from build123d import *

# Parameters (mm, degrees)
SKETCH_1_R               = 20
EXTRUDE_2_DEPTH          = 100
EXTRUDE_3_DEPTH          = 20
SKETCH_3_R               = 10.544762533
EXTRUDE_4_DEPTH          = 20
SKETCH_4_R               = 8
EXTRUDE_5_DEPTH          = 70
EXTRUDE_START            = 100
SKETCH_5_R               = 20
EXTRUDE_6_DEPTH          = 100
EXTRUDE_8_DEPTH          = 20
SKETCH_7_R               = 10.548482156
EXTRUDE_9_DEPTH          = 20
SKETCH_8_R               = 8
EXTRUDE_10_DEPTH         = 70
CUT_EXTRUDE_1_REACH      = 231.885
CUT_EXTRUDE_1_END_RADIUS = 20


with BuildPart() as part:
    # 草图1 → 凸台-拉伸2 (new body)
    with BuildSketch(Plane.XY):
        Circle(SKETCH_1_R)
    extrude(amount=EXTRUDE_2_DEPTH)

    # 草图2 → 凸台-拉伸3 (add)
    with BuildSketch(Plane.XY.offset(100)):
        Polygon((-20, 0), (-10.544762533, -101.307170503), (10.544762533, -101.307170503), (20, 0), align=None)
    extrude(amount=-EXTRUDE_3_DEPTH)

    # 草图3 → 凸台-拉伸4 (add, symmetric)
    with BuildSketch(Plane.XY.offset(100)):
        with Locations((0, -101.307170503)):
            Circle(SKETCH_3_R)
    extrude(amount=EXTRUDE_4_DEPTH, both=True)

    # 草图4 → 凸台-拉伸5 (add)
    with BuildSketch(Plane.XY.offset(120)):
        with Locations((0, -101.307170503)):
            Circle(SKETCH_4_R)
    extrude(amount=EXTRUDE_5_DEPTH)

    # 草图5 → 凸台-拉伸6 (add)
    with BuildSketch(Plane(origin=(0, 0, 0), x_dir=(-1, 0, 0), z_dir=(0, 0, -1)).offset(EXTRUDE_START)):
        Circle(SKETCH_5_R)
    extrude(amount=-EXTRUDE_6_DEPTH)

    # 草图6 → 凸台-拉伸8 (add)
    with BuildSketch(Plane(origin=(0, 0, -100), x_dir=(-1, 0, 0), z_dir=(0, 0, -1))):
        Polygon((20, 0), (10.548482156, 101.307517591), (-10.548482156, 101.307517591), (-20, 0), align=None)
    extrude(amount=-EXTRUDE_8_DEPTH)

    # 草图7 → 凸台-拉伸9 (add, symmetric)
    with BuildSketch(Plane(origin=(0, 0, -100), x_dir=(-1, 0, 0), z_dir=(0, 0, -1))):
        with Locations((0, 101.307517591)):
            Circle(SKETCH_7_R)
    extrude(amount=EXTRUDE_9_DEPTH, both=True)

    # 草图8 → 凸台-拉伸10 (add)
    with BuildSketch(Plane(origin=(0, 0, -120), x_dir=(-1, 0, 0), z_dir=(0, 0, -1))):
        with Locations((0, 101.307517591)):
            Circle(SKETCH_8_R)
    extrude(amount=EXTRUDE_10_DEPTH)

    # 切除-拉伸1: up to this cylinder (the profile starts inside it)
    cut_extrude_1_end = Plane(origin=(0, 0, 0), z_dir=(0, 0, -1)) * Cylinder(CUT_EXTRUDE_1_END_RADIUS, 504.77, mode=Mode.PRIVATE)
    # 草图9 → 切除-拉伸1 (cut, up to the surface)
    with BuildSketch(Plane(origin=(0, -16, 0), x_dir=(1, 0, 0), z_dir=(0, 1, 0)), mode=Mode.PRIVATE) as cut_extrude_1_sk1:
        with BuildLine():
            Line((6, -8), (6, 8))
            ThreePointArc((6, 8), (0, 14), (-6, 8))
            Line((-6, 8), (-6, -8))
            ThreePointArc((-6, -8), (0, -14), (6, -8))
        make_face()
    cut_extrude_1_tool1 = extrude(cut_extrude_1_sk1.sketch, amount=-CUT_EXTRUDE_1_REACH, mode=Mode.PRIVATE) & cut_extrude_1_end
    add(cut_extrude_1_tool1.solids().sort_by_distance((0, -16, 0))[0], mode=Mode.SUBTRACT)


solid = part.part
Source: CAD feature listing. Evaluate the final solid. Frame: model axes, mm. A direction names the side the tool comes from. Give positions to 0.01 mm unless a question says otherwise; leave off trailing zeros. Write each loop counter-clockwise with the first axis right and the second up, starting at its lowest first coordinate (ties: lowest second). Pieces come first, ordered by that corner, then holes. Notation, with made-up numbers: (-15.75, -0.5) -> (26.25, -0.5) arc R27 ccw to (26.25, 23.5) -> close; hole circle Ø2 at (24, 67.25). An arc over 180 degrees is marked (long way). Return JSON: item names as keys, results as strings. Group by question number.
1. Mould query, pull axis Z, two halves, no side actions, for faces 1 (the face through (0, -16, 0)), 2 (the face through (-2, -93, 120)), 3 (the face through (8, 104, -120)), 4 (the face through (1.373, 111.766, -104.724)). Classes: +Z half, -Z half, draft (parallel to the pull), parting line (faces both ways), or undercut.
2. Material intervals for line 1 (Z direction, x = 2, y = 38); line 2 (Y direction, x = 17, z = -7.5); line 3 (Z direction, x = 11, y = -48), sorted ascending. Write a range as from..to.
3. Pin query (flat end, axial travel): pin 1 Ø20 at (x, y) = (-1.5, 56.5) entering from -Z; pin 2 Ø10 at (x, z) = (13.5, 42.5) entering from -Y; pin 3 Ø2 at (x, y) = (3, 79.5) entering from +Z. Return the tip coordinate at first contact, or that it passes through.
4. Access query for faces 5 (the face through (1.04, 109.24, -154.51)), 6 (the face through (4.87, -110.66, 104.72)), 7 (the face through (0, 101, -190)). Directions: +Z, -Z, +X, -X, +Y, -Y. A direction counts if a zero-diameter tool reaches every point of the face in a straight line with its end or side. Return the directions, or none.
5. Section C-C, the plane y = -74. Output: boundary loops of the cut face in (x, z).
6. Section D-D, the plane z = 52. Output: boundary loops of the cut face in (x, y).
7. Section A-A, the plane x = 2. Output: boundary loops of the cut face in (y, z).
8. Section B-B, the plane z = -88.5. Output: boundary loops of the cut face in (x, y).
Determined:
{
 "1": {"face 1": "undercut", "face 2": "+Z half", "face 3": "-Z half", "face 4": "draft"},
 "2": {"line 1": "z = -100..-80", "line 2": "y = -10.54..10.54", "line 3": "z = 80..100"},
 "3": {"pin 1": "stops at z = -100", "pin 2": "stops at y = -18.1", "pin 3": "stops at z = -80"},
 "4": {"face 5": "-Z", "face 6": "+Z", "face 7": "-Z, +X, -X, +Y, -Y"},
 "5": {"outline": "(-13.09, 80) -> (13.09, 80) -> (13.09, 100) -> (-13.09, 100) -> close"},
 "6": {"outline": "circle Ø40 at (0, 0)"},
 "7": {"outline": "(-111.66, 80) -> (-19.9, 80) -> (-19.9, 13.66) -> (-16, 13.66) -> (-16, -13.66) -> (-19.9, -13.66) -> (-19.9, -100) -> (90.95, -100) -> (90.95, -120) -> (93.56, -120) -> (93.56, -190) -> (109.05, -190) -> (109.05, -120) -> (111.66, -120) -> (111.66, -80) -> (19.9, -80) -> (19.9, 100) -> (-90.95, 100) -> (-90.95, 120) -> (-93.56, 120) -> (-93.56, 190) -> (-109.05, 190) -> (-109.05, 120) -> (-111.66, 120) -> close"},
 "8": {"outline": "(-19.65, 3.7) arc R20 ccw (long way) to (19.65, 3.7) -> (10.55, 101.31) arc R10.55 ccw to (-10.55, 101.31) -> close"}
}
